Autodesk Inventor part; units mm, degrees
ref_plane "YZ Plane" through (0, 0, 0) normal (1, 0, 0) x (0, 1, 0)
ref_plane "XZ Plane" through (0, 0, 0) normal (0, 1, 0) x (-1, 0, 0)
ref_plane "XY Plane" through (0, 0, 0) normal (0, 0, 1) x (1, 0, 0)
sketch "Sketch1" plane through (0, 0, 0) normal (0, 1, 0) x (-1, 0, 0)
  line L0 (0, 0) -> (150, 0)
  line L1 (150, 0) -> (150, 150)
  line L2 (150, 150) -> (0, 150)
  line L3 (0, 150) -> (0, 0)
  dimension "d0" = 150
  dimension "d1" = 150
extrude "Extrusion1" add sketch "Sketch1" along normal blind 10
sketch "Sketch2" plane through (0, 10, 0) normal (0, 1, 0) x (1, 0, 0)
  line L0 (0, 0) -> (-150, 0)
  line L1 (-150, 0) -> (-146, 0)
  line L2 (-146, 0) -> (-146, -146)
  line L3 (-146, -146) -> (0, -146)
  line L4 (0, -150) -> (0, 0)
  line L5 (-150, 0) -> (-150, -150)
  line L6 (-150, -150) -> (0, -150)
  line L7 (0, -150) -> (0, 0)
  line L8 (0, 0) -> (-150, 0)
  dimension "d4" = 4
  dimension "d5" = 146
extrude "Extrusion2" add sketch "Sketch2" along normal blind 125 contours L2 L3 L4 L6 L5 L0
sketch "Sketch3" plane through (0, 0, 150) normal (1, 0, 0) x (0, 0, -1)
  line L0 (150, 0) -> (0, 0)
  line L1 (0, 0) -> (0, 5)
  line L2 (0, 0) -> (0, 135)
  line L3 (0, 5) -> (140, 5)
  line L4 (140, 5) -> (140, 0)
  line L5 (140, 0) -> (0, 0)
  dimension "d8" = 5
  dimension "d9" = 140
  dimension "d10" = 90
extrude "Extrusion3" add sketch "Sketch3" along normal blind 20
sketch "Sketch4" plane through (0, 0, 0) normal (0, 0, -1) x (-1, 0, 0)
  line L0 (150, 0) -> (-20, 0)
  line L1 (150, 0) -> (150, 5)
  line L2 (150, 5) -> (10, 5)
  line L3 (10, 5) -> (10, 0)
  line L4 (10, 0) -> (150, 0)
  point P0 (0, 0)
  point P1 (10, 0)
  dimension "d13" = 5
  dimension "d14" = 140
extrude "Extrusion4" cut sketch "Sketch4" against normal blind 20
sketch "Sketch5" plane through (0, 10, 146) normal (0, 0, -1) x (-1, 0, 0)
  line L0 (150, 125) -> (0, 125)
  line L1 (0, 125) -> (25, 125)
  line L2 (25, 125) -> (25, 85)
  line L3 (25, 85) -> (70, 85)
  line L4 (70, 85) -> (70, 28)
  line L5 (70, 28) -> (25, 28)
  line L6 (25, 28) -> (25, 85)
  line L7 (70, 85) -> (90, 85)
  line L8 (90, 85) -> (90, 28)
  line L9 (90, 28) -> (135, 28)
  line L10 (135, 28) -> (135, 85)
  line L11 (135, 85) -> (90, 85)
  line L12 (47.5, 85) -> (47.5, 80)
  line L13 (47.5, 80) -> (47.5, 33)
  line L14 (112.5, 85) -> (112.5, 80)
  line L15 (112.5, 80) -> (112.5, 33)
  point P0 (0, -10)
  dimension "d17" = 25
  dimension "d18" = 40
  dimension "d19" = 45
  dimension "d20" = 57
  dimension "d21" = 20
  dimension "d22" = 45
  dimension "d23" = 5
  dimension "d24" = 47
  dimension "d25" = 5
  dimension "d26" = 47
hole "Hole1" at (-47.5, 90, 146) at (-112.5, 90, 146) at (-112.5, 43, 146) at (-47.5, 43, 146) direction (0, 0, 1) diameter 4.318 end through all
sketch "Sketch6" plane through (-146, 10, 146) normal (1, 0, 0) x (0, 0, -1)
  line L0 (0, 125) -> (146, 125)
  line L1 (0, 125) -> (70, 125)
  line L2 (70, 125) -> (70, 85)
  line L3 (70, 85) -> (115, 85)
  line L4 (115, 85) -> (115, 28)
  line L5 (115, 28) -> (70, 28)
  line L6 (70, 28) -> (70, 85)
  line L7 (92.5, 85) -> (92.5, 80)
  line L8 (92.5, 80) -> (92.5, 33)
  point P0 (146, -10)
  dimension "d34" = 70
  dimension "d35" = 40
  dimension "d36" = 45
  dimension "d37" = 57
  dimension "d38" = 5
  dimension "d39" = 47
hole "Hole2" at (-146, 90, 53.5) at (-146, 43, 53.5) direction (-1, 0, 0) diameter 4.318 end through all
sketch "Sketch7" plane through (0, 0, 0) normal (0, -1, 0) x (1, 0, 0)
  line L0 (-150, 0) -> (-150, 150)
  line L1 (-150, 0) -> (-75, 0)
  line L2 (0, 0) -> (-146, 0)
  line L3 (-75, 0) -> (-75, 80)
  line L4 (-75, 80) -> (-55, 80)
  line L5 (-55, 80) -> (-95, 80)
  dimension "d47" = 75
  dimension "d48" = 80
  dimension "d49" = 20
  dimension "d50" = 40
hole "Hole3" at (-95, 0, 80) at (-55, 0, 80) direction (0, 1, 0) diameter 4 end through all counterbore diameter 6 counterbore depth 3
sketch "Sketch8" plane through (-150, 0, 150) normal (-1, 0, 0) x (0, 0, 1)
  line L0 (-150, 10) -> (-150, 135)
  line L1 (-150, 135) -> (-150, 125)
  line L2 (-150, 125) -> (-4, 125)
  line L3 (-4, 10) -> (-4, 135)
  line L4 (-4, 125) -> (-4, 120)
  line L5 (-4, 120) -> (-150, 120)
  line L6 (-150, 125) -> (-150, 120)
  point P0 (-150, 0)
  dimension "d58" = 10
  dimension "d59" = 146
  dimension "d60" = 5
extrude "Extrusion5" cut sketch "Sketch8" against normal blind 10
sketch "Sketch9" plane through (0, 10, 0) normal (0, 1, 0) x (1, 0, 0)
  line L0 (0, -10) -> (20, -10)
  line L1 (0, -10) -> (0, -55.3333)
  line L2 (0, -146) -> (0, 0)
  line L3 (0, -55.3333) -> (10, -55.3333)
  line L4 (10, -55.3333) -> (10, -100.6667)
  line L5 (-10, 0) -> (-10, -20)
  line L6 (-10, 0) -> (-55.3333, 0)
  line L7 (0, 0) -> (-146, 0)
  line L8 (-55.3333, 0) -> (-55.3333, -10)
  line L9 (-55.3333, -10) -> (-100.6667, -10)
  dimension "d63" = 45.3333
  dimension "d64" = 10
  dimension "d65" = 45.3333
  dimension "d66" = 45.3333
  dimension "d67" = 10
  dimension "d68" = 45.3333
hole "Hole4" at (10, 10, 100.6667) at (10, 10, 55.3333) at (-55.3333, 10, 10) at (-100.6667, 10, 10) direction (0, -1, 0) diameter 4.318 end through all
sketch "Sketch10" plane through (0, 10, 0) normal (0, 1, 0) x (1, 0, 0)
  point P0 (0, 0)
sketch "Sketch11" plane through (0, 0, 0) normal (0, -1, 0) x (1, 0, 0)
  circle A0 centre (10, 100.6667) radius 2.159
  circle A1 centre (10, 55.3333) radius 2.159
  circle A2 centre (-95, 80) radius 3
  circle A3 centre (-55, 80) radius 3
  line L0 (-10, 20) -> (-10, 0)
  line L1 (0, 0) -> (-10, 0)
  line L2 (0, 10) -> (0, 0)
  line L3 (0, 10) -> (20, 10)
  line L4 (20, 150) -> (20, 10)
  line L5 (-150, 150) -> (20, 150)
  line L6 (-150, 20) -> (-150, 150)
  line L7 (-150, 20) -> (-10, 20)
extrude "Extrusion6" add sketch "Sketch11" along normal blind 3
sketch "Sketch12" plane through (-55, 3, 80) normal (0, -1, 0) x (1, 0, 0)
  circle A0 centre (0, 0) radius 3
  circle A1 centre (0, 0) radius 2
  circle A2 centre (-40, 0) radius 3
  circle A3 centre (-40, 0) radius 2
  point P0 (55, -80)
extrude "Extrusion7" add sketch "Sketch12" along normal blind 3
sketch "Sketch13" plane through (0, -3, 0) normal (0, -1, 0) x (1, 0, 0)
  circle A0 centre (10, 100.6667) radius 2.159
  circle A1 centre (10, 55.3333) radius 2.159
  point P0 (0, 0)
hole "Hole5" at (10, -3, 100.6667) at (10, -3, 55.3333) direction (0, 1, 0) diameter 4.318 end through all counterbore diameter 7.62 counterbore depth 5.08
properties part number "Quarter 2"
Model file for the job. Use its own axes, mm. A direction names the side the tool comes from. Round coordinates to 2 decimals unless told otherwise and drop trailing zeros. Order: outer loops, then holes, each group sorted by start corner. A loop starts at its lowest first (then second) coordinate and runs counter-clockwise, first axis right, second up.
(1) 3-axis set-ups, long thin cutter, end or side, ignore diameter. For faces 1 (the face through (-93, 0, 79)), 2 (the face through (10, 1, 10)), 3 (the face through (-81, 5, 10)), 4 (the face through (-72, 10, 74)): which of +Z, -Z, +X, -X, +Y, -Y reach the whole face in a straight line?
(2) Band-saw the part on A-A (z = 27). List the corners of the cut face in (x, y).
(3) Drill centre lines: line 1 (X direction, y = 8.25, z = 80); line 2 (X direction, y = 43, z = 149); line 3 (Z direction, x = -55, y = 6). Where is each one in solid material? Low to high.
(4) Band-saw the part on B-B (y = 90). List the corners of the cut face in (x, z).
(5) Band-saw the part on C-C (x = -120.5). List the corners of the cut face in (y, z).
(6) Pin check, flat tips, straight feed: pin 1 (10 mm diameter, centred on x = 5.5, z = 87, fed in from +Y); pin 2 (7 mm diameter, centred on x = 10, z = 55.33, fed in from -Y); pin 3 (4 mm diameter, centred on x = -35.5, y = 26, fed in from -Z). Stop position of each tip, or through.
(7) Band-saw the part on D-D (y = 70). List the corners of the cut face in (x, z).
(8) Pull direction Y, two halves, no side cores. Call faces 5 (the face through (-109, 135, 147)), 6 (the face through (-148.03, 88.18, 52.34)), 7 (the face through (12, 2.08, 54)): released by +Y, released by -Y, zero draft, split by the parting line, or undercut.
Verdict:
1. face 1: -Y
1. face 2: -Z, +X, +Y, -Y
1. face 3: -Z, -X, -Y
1. face 4: -Z, +X, +Y
2. outline: (-150, -3) - (20, -3) - (20, 5) - (0, 5) - (0, 10) - (-146, 10) - (-146, 120) - (-150, 120) - close; (-150, 125) - (-146, 125) - (-146, 135) - (-150, 135) - close
3. line 1: x = -150 to -97, -93 to -57, -53 to 0
3. line 2: x = -150 to -114.66, -110.34 to -49.66, -45.34 to 0
3. line 3: z = 0 to 7.87, 12.13 to 78, 82 to 150
4. outline: (-150, 0) - (-146, 0) - (-146, 51.34) - (-150, 51.34) - close; (-150, 55.66) - (-146, 55.66) - (-146, 146) - (-114.66, 146) - (-114.66, 150) - (-150, 150) - close; (-110.34, 146) - (-49.66, 146) - (-49.66, 150) - (-110.34, 150) - close; (-45.34, 146) - (0, 146) - (0, 150) - (-45.34, 150) - close
5. outline: (-3, 20) - (5, 20) - (5, 0) - (10, 0) - (10, 146) - (135, 146) - (135, 150) - (-3, 150) - close
6. pin 1: stops at y = 5
6. pin 2: stops at y = 2.08
6. pin 3: stops at z = 146
7. outline: (-150, 0) - (-146, 0) - (-146, 146) - (0, 146) - (0, 150) - (-150, 150) - close
8. face 5: released by +Y
8. face 6: undercut
8. face 7: released by -Y
